Geometry: see drawing. Coordinates: mm, zero at the bounding-box minimum. A direction names the side the tool comes from. Round coordinates to 2 decimals unless told otherwise and drop trailing zeros. Write each loop counter-clockwise with the first axis right and the second up, starting at its lowest first coordinate (ties: lowest second). Pieces come first, ordered by that corner, then holes.
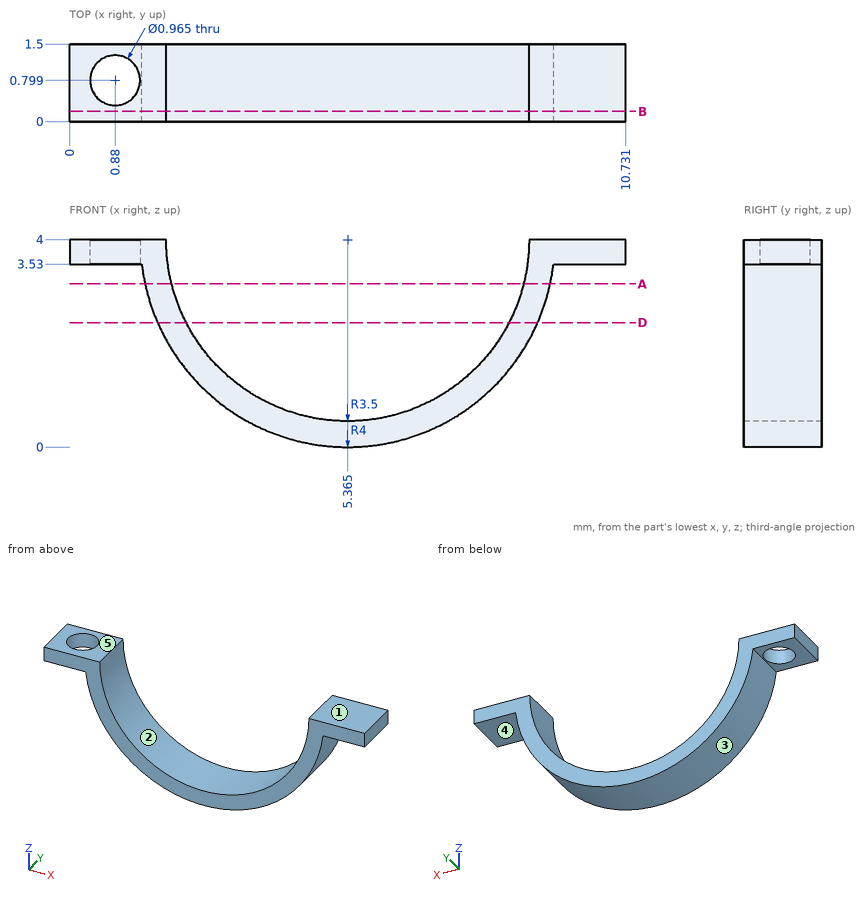
1) Contact query for flat-ended pins moving along their axis: P1, Ø0.7, axis at x = 10.5, y = 0.5, coming from the -Z side; P2, Ø2, axis at x = 5.5, z = 2, coming from the +Y side. Output: stop coordinate, or through.
Taken from the geometry:
P1: stops at z = 3.53
P2: passes through
2) Section query A-A on z = 3.15. Return the cut outline in (x, y) (1 decimal).
Taken from the geometry:
outline: (1.5, 0) - (2, 0) - (2, 1.5) - (1.5, 1.5) - close; (8.8, 0) - (9.3, 0) - (9.3, 1.5) - (8.8, 1.5) - close
3) Section query B-B on y = 0.2. Return the cut outline in (x, z) (1 decimal).
Taken from the geometry:
outline: (0, 3.5) - (1.4, 3.5) arc R4 ccw to (9.3, 3.5) - (10.7, 3.5) - (10.7, 4) - (8.9, 4) arc R3.5 cw to (1.9, 4) - (0, 4) - close
4) Pull-direction query (X, two-part tool) for the marked faces 1, 2 and 3; classes: released by +X, released by -X, zero draft, split by the parting line, or undercut.
Taken from the geometry:
face 1: zero draft
face 2: undercut
face 3: split by the parting line
5) Section query D-D on z = 2.4. Return the cut outline in (x, y).
Taken from the geometry:
outline: (1.7, 0) - (2.25, 0) - (2.25, 1.5) - (1.7, 1.5) - close; (8.48, 0) - (9.03, 0) - (9.03, 1.5) - (8.48, 1.5) - close
6) Material intervals for line 1 (X direction, y = 0.45, z = 1.65) (1 decimal); line 2 (Z direction, x = 10.25, y = 0.3); line 3 (X direction, y = 0.55, z = 3.3) (1 decimal), sorted ascending.
Taken from the geometry:
line 1: x = 2.1 to 2.8, 8 to 8.6
line 2: z = 3.53 to 4
line 3: x = 1.4 to 1.9, 8.8 to 9.3
7) Reachability of the marked faces 4 and 5 from +Z, -Z, +X, -X, +Y, -Y: full face, straight path, thin tool, end or side. Return the list, or none.
Taken from the geometry:
face 4: -Z, +X, +Y, -Y
face 5: +Z, +X, -X, +Y, -Y
